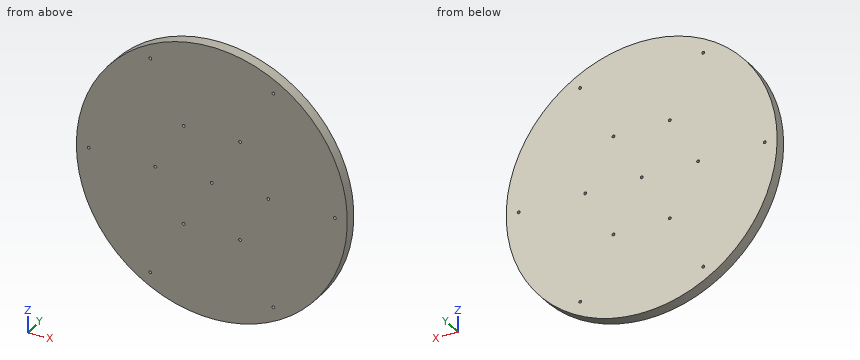
Autodesk Inventor part; units mm, degrees
ref_plane "YZ Plane" through (0, 0, 0) normal (1, 0, 0) x (0, 1, 0)
ref_plane "XZ Plane" through (0, 0, 0) normal (0, 1, 0) x (-1, 0, 0)
ref_plane "XY Plane" through (0, 0, 0) normal (0, 0, 1) x (1, 0, 0)
sketch "Sketch1" plane through (0, 0, 0) normal (0, 1, 0) x (-1, 0, 0)
  circle A0 centre (0.7015, 0) radius 305
  point P0 (0, 0)
  dimension "d0" = 610
extrude "Extrusion1" add sketch "Sketch1" along normal blind 25.4
sketch "Sketch2" plane through (-0.7015, 25.4, 0) normal (0, 1, 0) x (1, 0, 0)
  circle A0 centre (0, 0) radius 305
  circle A1 centre (0, 0) radius 4.5
  circle A2 centre (127, 0) radius 4.5
  circle A3 centre (277, 0) radius 4.5
  dimension "d3" = 127
  dimension "d4" = 150
  dimension "d15" = 9
  dimension "d16" = 9
  dimension "d17" = 9
hole "Hole1" at (-0.7015, 25.4, 0) at (126.2985, 25.4, 0) at (276.2985, 25.4, 0) direction (0, -1, 0) diameter 6.35 end through all
pattern_circular "Circular Pattern1" count 6 over 360 about axis through (-0.7015, -837.6441, 0) along (0, 1, 0) of "Hole1"
properties part number "bpSparJig" material "Wood (Cherry)"
Geometry: final body of the model. Coordinates: model frame, mm. Round coordinates to 2 decimals unless told otherwise and drop trailing zeros. Loops run counter-clockwise (first coordinate to the right, second up) from the corner with the lowest first, then second, coordinate; pieces in that order, holes last.
Q1. Material intervals for L1, parallel to X at y = 23, z = 51.5; L2, parallel to Z at x = -162.5, y = 8.75; L3, parallel to X at y = 23.25, z = -163, sorted ascending.
Q2. Pin query (flat end, axial travel): P1, Ø10, axis at x = -43, y = 4, coming from the -Z side; P2, Ø12, axis at y = 8.5, z = -172, coming from the -X side; P3, Ø5, axis at x = -134.5, y = 17, coming from the +Z side. Return the tip coordinate at first contact, or that it passes through.
Q3. Section A-A on y = 14.5. State how many separate pieces and enclosed holes the cut face has, plus the area to 3 significant figures.
Q4. Section B-B on z = 211. Return loops of the section in (x, y).
Q5. Section C-C on x = -254. Return loops of the section in (y, z), plus the area to 3 significant figures.
Evaluation:
1. L1: x = -301.32 to 299.92
1. L2: z = -258.55 to 258.55
1. L3: x = -258.49 to 257.09
2. P1: stops at z = -302.71
2. P2: stops at x = -256.57
2. P3: stops at z = 275.29
3. separate pieces: 1
3. enclosed holes: 13
3. area: 292,000 mm2
4. outline: (-220.94, 0) - (219.53, 0) - (219.53, 25.4) - (-220.94, 25.4) - close
5. outline: (0, -169.9) - (25.4, -169.9) - (25.4, 169.9) - (0, 169.9) - close
5. area: 8,630 mm2
